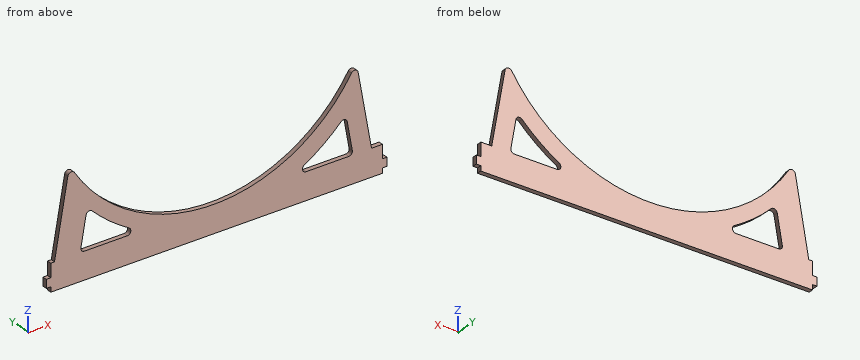
```python
from build123d import *

# Parameters (mm, degrees)
SKETCH1_W               = 666.75
SKETCH1_H               = 19.05
BOSS_EXTRUDE1_DEPTH     = 3.175
SKETCH2_W               = 3.175
SKETCH2_H               = 9.525
CUT_EXTRUDE2_DEPTH      = 334.526156208
TOP_BALL_SECURING_DEPTH = 3.175
FILLET2_R               = 2.54
CUT_EXTRUDE3_DEPTH      = 340.618903378
CUT_EXTRUDE8_REACH      = 341.619
SKETCH12_W              = 214.0585
SKETCH12_H              = 19.05
CUT_EXTRUDE9_REACH      = 137.789
SKETCH13_W              = 3.175
SKETCH13_H              = 3.53251897


with BuildPart() as part:
    # Sketch1 → Boss-Extrude1 (new body)
    with BuildSketch(Plane(origin=(0, 0, 0), x_dir=(1, 0, 0), z_dir=(0, 1, 0))):
        Rectangle(SKETCH1_W, SKETCH1_H)
    extrude(amount=BOSS_EXTRUDE1_DEPTH)

    # Sketch2 → Cut-Extrude2 (cut, through all)
    with BuildSketch(Plane.XZ):
        with Locations((-331.7875, 4.7625)):
            Rectangle(SKETCH2_W, SKETCH2_H)
        with Locations((-117.729, 4.7625)):
            Rectangle(SKETCH2_W, SKETCH2_H)
    cut_extrude2 = extrude(amount=-CUT_EXTRUDE2_DEPTH, mode=Mode.SUBTRACT)

    # Mirror1: Cut-Extrude2 across plane
    add(cut_extrude2.mirror(Plane(origin=(0, 0, 0), x_dir=(0, 0, 1), z_dir=(1, 0, 0))), mode=Mode.SUBTRACT)

    # Sketch3 → top ball securing (add)
    with BuildSketch(Plane(origin=(0, 3.175, 0), x_dir=(1, 0, 0), z_dir=(0, 1, 0))):
        with BuildLine():
            Line((108.470225533, -9.525), (97.899375359, -69.475270408))
            ThreePointArc((97.899375359, -69.475270408), (-2.54, -9.731863753), (-102.979375359, -69.475270408))
            Line((-102.979375359, -69.475270408), (-113.550225533, -9.525))
            Line((-113.550225533, -9.525), (108.470225533, -9.525))
        make_face()
    extrude(amount=-TOP_BALL_SECURING_DEPTH)

    # Fillet2
    fillet2_edges = [part.edges().sort_by_distance(p)[0] for p in [
        (-102.979375359, 1.5875, 69.475270408),
        (97.899375359, 1.5875, 69.475270408),
    ]]
    fillet(fillet2_edges, radius=FILLET2_R)

    # Sketch5 → Cut-Extrude3 (cut, through all)
    with BuildSketch(Plane(origin=(0, 3.175, 0), x_dir=(1, 0, 0), z_dir=(0, 1, 0))):
        with BuildLine():
            Line((-91.472594393, -32.786971326), (-95.048665129, -12.506066371))
            ThreePointArc((-95.048665129, -12.506066371), (-94.493006322, -10.432319471), (-92.547253437, -9.525))
            Line((-92.547253437, -9.525), (-62.60624334, -9.525))
            ThreePointArc((-62.60624334, -9.525), (-60.153898656, -11.403482389), (-61.32886602, -14.260428701))
            ThreePointArc((-61.32886602, -14.260428701), (-74.893704079, -23.368953639), (-87.176845785, -34.143668852))
            ThreePointArc((-87.176845785, -34.143668852), (-89.736130888, -34.767981392), (-91.472594393, -32.786971326))
        make_face()
        with BuildLine():
            Line((92.547253437, -9.525), (62.60624334, -9.525))
            ThreePointArc((62.60624334, -9.525), (60.153898656, -11.403482389), (61.32886602, -14.260428701))
            ThreePointArc((61.32886602, -14.260428701), (74.893704079, -23.368953639), (87.176845785, -34.143668852))
            ThreePointArc((87.176845785, -34.143668852), (89.736130888, -34.767981392), (91.472594393, -32.786971326))
            Line((91.472594393, -32.786971326), (95.048665129, -12.506066371))
            ThreePointArc((95.048665129, -12.506066371), (94.493006322, -10.432319471), (92.547253437, -9.525))
        make_face()
    extrude(amount=-CUT_EXTRUDE3_DEPTH, mode=Mode.SUBTRACT)

    # Sketch12 → Cut-Extrude8 (cut, up to next)
    with BuildSketch(Plane.XZ, mode=Mode.PRIVATE) as cut_extrude8_sk1:
        with Locations((226.34575, 0)):
            Rectangle(SKETCH12_W, SKETCH12_H)
    cut_extrude8_tool1 = extrude(cut_extrude8_sk1.sketch, amount=-CUT_EXTRUDE8_REACH, mode=Mode.PRIVATE) & part.part
    # Sketch12 → Cut-Extrude8 (cut, up to next)
    with BuildSketch(Plane.XZ, mode=Mode.PRIVATE) as cut_extrude8_sk2:
        with Locations((-226.34575, 0)):
            Rectangle(SKETCH12_W, SKETCH12_H)
    cut_extrude8_tool2 = extrude(cut_extrude8_sk2.sketch, amount=-CUT_EXTRUDE8_REACH, mode=Mode.PRIVATE) & part.part
    add(cut_extrude8_tool1.solids().sort_by_distance((226.34575, 0, 0))[0], mode=Mode.SUBTRACT)
    add(cut_extrude8_tool2.solids().sort_by_distance((-226.34575, 0, 0))[0], mode=Mode.SUBTRACT)

    # Sketch13 → Cut-Extrude9 (cut, up to next)
    with BuildSketch(Plane.XZ, mode=Mode.PRIVATE) as cut_extrude9_sk1:
        with Locations((117.729, -7.758740515)):
            Rectangle(SKETCH13_W, SKETCH13_H)
    cut_extrude9_tool1 = extrude(cut_extrude9_sk1.sketch, amount=-CUT_EXTRUDE9_REACH, mode=Mode.PRIVATE) & part.part
    # Sketch13 → Cut-Extrude9 (cut, up to next)
    with BuildSketch(Plane.XZ, mode=Mode.PRIVATE) as cut_extrude9_sk2:
        with Locations((-117.729, -7.758740515)):
            Rectangle(SKETCH13_W, SKETCH13_H)
    cut_extrude9_tool2 = extrude(cut_extrude9_sk2.sketch, amount=-CUT_EXTRUDE9_REACH, mode=Mode.PRIVATE) & part.part
    add(cut_extrude9_tool1.solids().sort_by_distance((117.729, 0, -7.758741))[0], mode=Mode.SUBTRACT)
    add(cut_extrude9_tool2.solids().sort_by_distance((-117.729, 0, -7.758741))[0], mode=Mode.SUBTRACT)


solid = part.part
```
For this review, take the finished solid that the model builds, in its own axes (mm). Give positions to 0.01 mm unless a question says otherwise; leave off trailing zeros. Order: outer loops, then holes, each group sorted by start corner. A loop starts at its lowest first (then second) coordinate and runs counter-clockwise, first axis right, second up.
1) Take a section at A-A (y = 1.6). State how many separate pieces and enclosed holes the cut face has, then the cut area to 3 significant figures.
2) Insertion check: pin 1 (1 mm diameter, centred on x = -75.5, y = 1, fed in from +Z); pin 2 (1 mm diameter, centred on x = 118.5, y = 1.5, fed in from -Z); pin 3 (2 mm diameter, centred on x = -74, z = 31, fed in from -Y); pin 4 (1 mm diameter, centred on x = -118, y = 2, fed in from +Z). Each pin has a flat end and moves straight along its axis. Give the tip position at first contact, or say it passes through.
3) Wall thickness on line 1 (X direction, y = 1.1, z = 23); line 2 (X direction, y = 2.85, z = 19); line 3 (X direction, y = 2.45, z = 8): over which ranges is each line inside the solid? List them lowest first.
4) Take a section at C-C (z = 21.5). Give the boundary of the cut face in (x, y) (3 decimals).
5) Take a section at B-B (x = 75.5). Give the boundary of the cut face in (y, z) (3 decimals).
6) Take a section at D-D (z = 41). Give the boundary of the cut face in (x, y) (3 decimals), then the cut area to 3 significant figures.
Derived:
1. separate pieces: 1
1. enclosed holes: 2
1. area: 7,550 mm2
2. pin 1: stops at z = 36.46
2. pin 2: stops at z = -5.99
2. pin 3: stops at y = 0
2. pin 4: stops at z = 0
3. line 1: x = -111.17 to -93.2, -74.41 to -55.99, 50.91 to 74.41, 93.2 to 106.09
3. line 2: x = -111.88 to -93.9, -68.86 to -47.63, 42.55 to 68.86, 93.9 to 106.8
3. line 3: x = -116.14 to 116.14
4. outline: (-111.439, 0) - (-93.463, 0) - (-93.463, 3.175) - (-111.439, 3.175) - close; (-72.401, 0) - (-53.054, 0) - (-53.054, 3.175) - (-72.401, 3.175) - close; (47.974, 0) - (72.401, 0) - (72.401, 3.175) - (47.974, 3.175) - close; (93.463, 0) - (106.359, 0) - (106.359, 3.175) - (93.463, 3.175) - close
5. outline: (0, -9.525) - (3.175, -9.525) - (3.175, 9.525) - (0, 9.525) - close; (0, 23.838) - (3.175, 23.838) - (3.175, 40.52) - (0, 40.52) - close
6. outline: (-108, 0) - (-81.091, 0) - (-81.091, 3.175) - (-108, 3.175) - close; (76.011, 0) - (102.92, 0) - (102.92, 3.175) - (76.011, 3.175) - close
6. area: 171 mm2
